Job drawing, mm, ordinate dimensions from the low corner. One solid piece. Coordinates: 2 decimals unless noted, no trailing zeros. Loops run counter-clockwise (first coordinate to the right, second up) from the corner with the lowest first, then second, coordinate; pieces in that order, holes last. Notation, with made-up numbers: (-15.75, 86) - (-11.75, 86) arc R18 ccw to (-11.75, 93) - close; hole circle Ø1 at (-3.5, 0.5). An arc over 180 degrees is marked (long way). Use a Markdown table: item, result. Add a question column.
1. Drop a flat-ended pin along its axis: pin 1 (1 mm diameter, centred on x = 54, z = 3, fed in from -Y). Give the stop position or say it passes through.
2. Wall check: probe 1 along Y at (x, z) = (60.5, 4.75); probe 2 along X at (y, z) = (103.5, 1.5); probe 3 along X at (y, z) = (80.5, 4.25). Give the ranges that are in metal, low to high. Write a range as [from, to].
3. Band-saw the part on B-B, the plane z = 4. Give the cut face in (x, y) (3 decimals).
4. Band-saw the part on A-A, the plane y = 88.9. Give the cut face in (x, z).
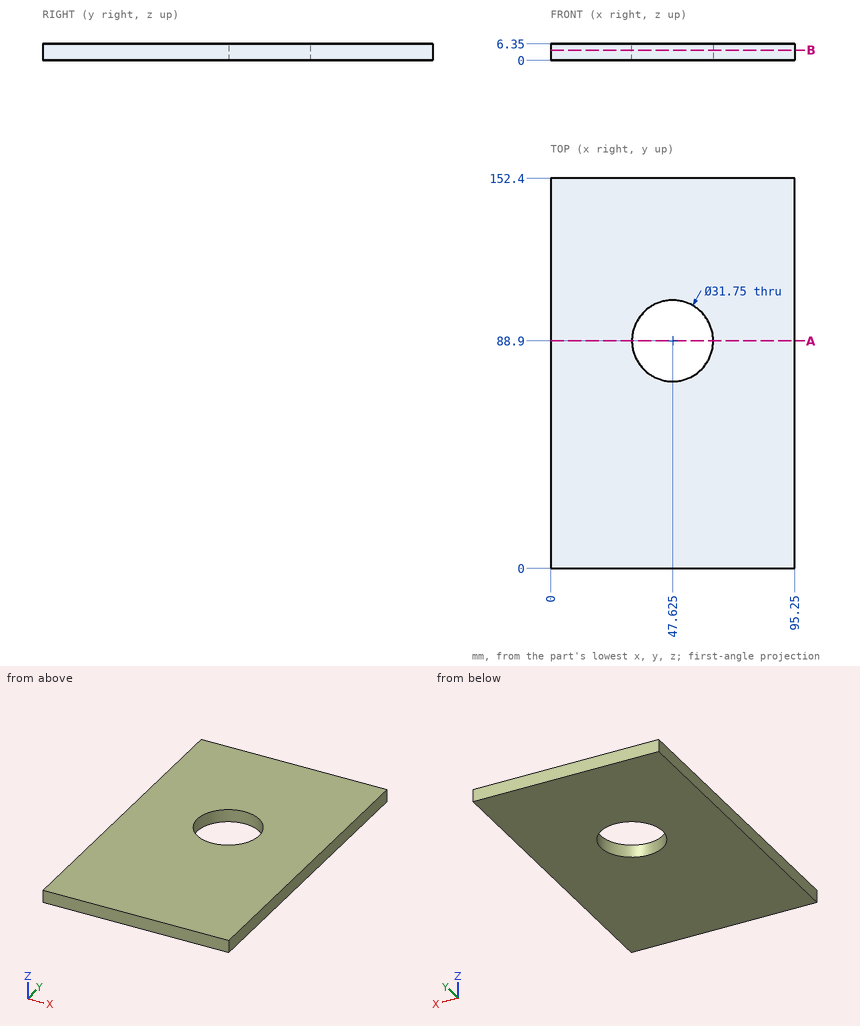
Geometry check:
| question | item | result |
|---|---|---|
| 1 | pin 1 | stops at y = 0 |
| 2 | probe 1 | y = [0, 79.61], [98.19, 152.4] |
| 2 | probe 2 | x = [0, 41.39], [53.86, 95.25] |
| 2 | probe 3 | x = [0, 34.15], [61.1, 95.25] |
| 3 | outline | (0, 0) - (95.25, 0) - (95.25, 152.4) - (0, 152.4) - close; hole circle Ø31.75 at (47.625, 88.9) |
| 4 | outline | (0, 0) - (31.75, 0) - (31.75, 6.35) - (0, 6.35) - close; (63.5, 0) - (95.25, 0) - (95.25, 6.35) - (63.5, 6.35) - close |
